```python
from build123d import *

# Parameters (mm, degrees)
SKETCH2_W           = 68.58
SKETCH2_H           = 24.13
SKETCH2_R           = 2.6
BOSS_EXTRUDE1_DEPTH = 6.35
CUT_EXTRUDE1_DEPTH  = 7.35
FILLET3_R           = 2.54


with BuildPart() as part:
    # Sketch2 → Boss-Extrude1 (new body)
    with BuildSketch(Plane(origin=(0, 0, 0), x_dir=(1, 0, 0), z_dir=(0, 1, 0))):
        with Locations((34.29, 12.065)):
            Rectangle(SKETCH2_W, SKETCH2_H)
        with Locations((4.57, 12.065)):
            Circle(SKETCH2_R, mode=Mode.SUBTRACT)
        with Locations((64.01, 12.065)):
            Circle(SKETCH2_R, mode=Mode.SUBTRACT)
    extrude(amount=BOSS_EXTRUDE1_DEPTH)

    # Sketch3 → Cut-Extrude1 (cut, through all)
    with BuildSketch(Plane(origin=(0, 6.35, 0), x_dir=(1, 0, 0), z_dir=(0, 1, 0))):
        with BuildLine():
            Line((4.57, 3.715), (0, 3.715))
            Line((0, 3.715), (0, 0))
            Line((0, 0), (6.57, 0))
            Line((6.57, 0), (6.57, 1.715))
            ThreePointArc((6.57, 1.715), (5.984213562, 3.129213562), (4.57, 3.715))
        make_face()
        with BuildLine():
            ThreePointArc((4.57, 20.415), (5.984213562, 21.000786438), (6.57, 22.415))
            Line((6.57, 22.415), (6.57, 24.13))
            Line((6.57, 24.13), (0, 24.13))
            Line((0, 24.13), (0, 20.415))
            Line((0, 20.415), (4.57, 20.415))
        make_face()
    extrude(amount=-CUT_EXTRUDE1_DEPTH, mode=Mode.SUBTRACT)

    # Fillet3
    fillet3_edges = [part.edges().sort_by_distance(p)[0] for p in [
        (6.57, 3.175, 0),
        (0, 3.175, -3.715),
        (0, 3.175, -20.415),
        (6.57, 3.175, -24.13),
    ]]
    fillet(fillet3_edges, radius=FILLET3_R)


solid = part.part
```
Can you work these out from the model? Positions are in its coordinate system, mm. A direction names the side the tool comes from. Coordinates: 2 decimals unless noted, no trailing zeros. Loops run counter-clockwise (first coordinate to the right, second up) from the corner with the lowest first, then second, coordinate; pieces in that order, holes last. Notation, with made-up numbers: (86.25, 1) - (125.25, 1) arc R27 ccw to (125.25, 31) - close; hole circle Ø3 at (2.25, 51.5). An arc over 180 degrees is marked (long way). Answer as CSV lines item,"result". Start each with the question number.
1) Suppose I cut it at B-B (y = 3). Count the separate pieces of the cut face and the enclosed holes in it, plus the area to 3 significant figures.
2) Which directions (+Z, -Z, +X, -X, +Y, -Y) give clear straight access to the entire face, cutting with the end or side of a thin tool? Please do faces 5 (the flat face through (0, 3, -12)), 6 (the flat face through (4, 3, -20.415)), 7 (the flat face through (4, 3, -3.715)).
3) For pin 1 (8.5 mm diameter, centred on x = 64.01, z = -12.065, fed in from +Y); pin 2 (0.6 mm diameter, centred on x = 3.5, y = 2.5, fed in from -Z) (3 decimals); pin 3 (0.6 mm diameter, centred on x = 3, y = 4.5, fed in from +Z) (3 decimals), each with a flat end and sliding along its axis, tell me the tip position at first contact or that it passes through.
4) Suppose I cut it at A-A (x = 64.01). Please give me the cut outline in (y, z) (3 decimals).
5) I need wall thicknesses on line 1 (Z direction, x = 64.01, y = 2) (3 decimals); line 2 (Z direction, x = 4.57, y = 3.25) (3 decimals); line 3 (X direction, y = 3, z = -10). Which ranges of each line are inside material? Lowest first, please. Write a range as from..to.
6) Thinking about a two-plate mould opening in Z: for faces 1 (the cylindrical face through (4.232, 3.131, -14.643)), 2 (the flat face through (38, 3, -24.13)), 3 (the cylindrical face through (65.408, 3.131, -14.257)), 4 (the flat face through (68.58, 3, -12)), which applies, pulls with the +Z half, pulls with the -Z half, needs draft (parallel to the pull), parting line crosses it, or undercut?
Check result:
1,separate pieces,"1"
1,enclosed holes,"2"
1,area,"1,560 mm²"
2,face 5,"+Z, -Z, -X, +Y, -Y"
2,face 6,"-Z, -X, +Y, -Y"
2,face 7,"+Z, -X, +Y, -Y"
3,pin 1,"stops at y = 6.35"
3,pin 2,"stops at z = -20.415"
3,pin 3,"stops at z = -3.715"
4,outline,"(0, -24.13) - (6.35, -24.13) - (6.35, -14.665) - (0, -14.665) - close; (0, -9.465) - (6.35, -9.465) - (6.35, 0) - (0, 0) - close"
5,line 1,"z = -24.13..-14.665, -9.465..0"
5,line 2,"z = -20.415..-14.665, -9.465..-3.715"
5,line 3,"x = 0..2.99, 6.15..62.43, 65.59..68.58"
6,face 1,"undercut"
6,face 2,"pulls with the -Z half"
6,face 3,"undercut"
6,face 4,"needs draft"
